from build123d import *

# Parameters (mm, degrees)
F1_DEPTH   = 12.7
F1_FACE1_W = 781.05
F1_FACE1_H = 12.7
F4_SIZE    = 6.35
F6_D       = 19.05
F6_DEPTH   = 1524
F6_TIP     = 5.7231973962


with BuildPart() as f1:
    # F0 (on Front) → F1 (new body)
    with BuildSketch(Plane.XZ):
        Polygon((-307.975, -336.55), (-307.975, -381), (307.975, -381), (307.975, -336.55), (390.525, -336.55), (390.525, 381), (-390.525, 381), (-390.525, -336.55), align=None)
    extrude(amount=F1_DEPTH)

    # F3: sweep along a path in F2
    with BuildLine(Plane(origin=(-390.525, 0, 0), x_dir=(0, -1, 0), z_dir=(-1, 0, 0))) as f3_path:
        Line((6.35, 381), (24.3105122421, 398.9605122421))
        Line((24.3105122421, 398.9605122421), (78.2855122421, 398.9605122421))
    # F1_face1 (on face) → F3 (sweep)
    with BuildSketch(Plane(origin=(0, -6.35, 381), x_dir=(1, 0, 0), z_dir=(0, 0, 1))):
        Rectangle(F1_FACE1_W, F1_FACE1_H)
    sweep(path=f3_path.line, transition=Transition.RIGHT)

    # F4
    f4_edges = [f1.edges().sort_by_distance(p)[0] for p in [
        (-390.525, -78.285512, 398.960512),
        (390.525, -78.285512, 398.960512),
    ]]
    chamfer(f4_edges, length=F4_SIZE)

    # F6
    with Locations(Plane.XY.offset(403.4506403027)):
        with Locations((0, -38.8703841816)):
            Hole(F6_D / 2, depth=F6_DEPTH)
            with Locations((0, 0, -(F6_DEPTH + F6_TIP / 2))):  # 118° drill point
                Cone(0, F6_D / 2, F6_TIP, mode=Mode.SUBTRACT)


solid = f1.part
Geometry: final body of the model. Coordinates: model frame, mm. A direction names the side the tool comes from. Coordinates: 2 decimals unless noted, no trailing zeros. Write each loop counter-clockwise with the first axis right and the second up, starting at its lowest first coordinate (ties: lowest second). Pieces come first, ordered by that corner, then holes. Notation, with made-up numbers: (11.25, -16) - (16.25, -16) arc R18 ccw to (16.25, -1) - close; hole circle Ø1 at (-27.75, 37). An arc over 180 degrees is marked (long way). Return JSON: item names as keys, results as strings.
Item 1: Section query B-B (x = -259.5). Output: boundary loops of the cut face in (y, z), and give its area (3 significant figures).
Completed:
{"outline": "(-82.78, 394.47) - (-26.17, 394.47) - (-12.7, 381) - (-12.7, -381) - (0, -381) - (0, 381) - (-22.45, 403.45) - (-73.8, 403.45) - close", "area": "10,400 mm2"}
Item 2: Section query A-A (x = 0). Output: boundary loops of the cut face in (y, z), and give its area (3 significant figures).
Completed:
{"outline": "(-82.78, 394.47) - (-48.4, 394.47) - (-48.4, 403.45) - (-73.8, 403.45) - close; (-29.35, 394.47) - (-26.17, 394.47) - (-12.7, 381) - (-12.7, -381) - (0, -381) - (0, 381) - (-22.45, 403.45) - (-29.35, 403.45) - close", "area": "10,200 mm2"}
Item 3: Pull-direction query (Y, two-part tool) for faces 3 (the face through (2.06, -48.17, 398.9)), 4 (the face through (-5, -12.7, 5)), 5 (the face through (5, -48, 403.451)), 6 (the face through (5, -11, 392)); classes: +Y half, -Y half, draft (parallel to the pull), parting line (faces both ways), or undercut.
Completed:
{"face 3": "undercut", "face 4": "-Y half", "face 5": "draft", "face 6": "+Y half"}
Item 4: Pin query (flat end, axial travel): pin 1 Ø10 at (x, y) = (357, -8) entering from -Z; pin 2 Ø8 at (x, z) = (-174.5, -171.5) entering from -Y; pin 3 Ø4 at (y, z) = (-6, -366.5) entering from +X (3 decimals). Return the tip coordinate at first contact, or that it passes through.
Completed:
{"pin 1": "stops at z = -336.55", "pin 2": "stops at y = -12.7", "pin 3": "stops at x = 307.975"}
Item 5: Reachability of faces 1 (the face through (-5, 0, 5)), 2 (the face through (-5, -55, 394.47)) from +Z, -Z, +X, -X, +Y, -Y: full face, straight path, thin tool, end or side. Return the list, or none.
Completed:
{"face 1": "+Z, -Z, +X, -X, +Y", "face 2": "-Z, +X, -X, -Y"}
Item 6: Section query C-C (z = 310.5). Output: boundary loops of the cut face in (x, y) (3 decimals).
Completed:
{"outline": "(-390.525, -12.7) - (390.525, -12.7) - (390.525, 0) - (-390.525, 0) - close"}
Item 7: Line query: L1, parallel to Y at x = -279, z = -15; L2, parallel to Z at x = 138, y = -61.5; L3, parallel to Y at x = 0, z = 399.75. Output: solid intervals per line, ascending.
Completed:
{"L1": "y = -12.7 to 0", "L2": "z = 394.47 to 403.45", "L3": "y = -77.5 to -48.4, -29.35 to -18.75"}
